Build history of the part. All positions in model axes, mm. Face numbers are marked on the shaded views. A direction names the side the tool comes from. Give positions to 0.01 mm unless a question says otherwise; leave off trailing zeros. Order: outer loops, then holes, each group sorted by start corner. A loop starts at its lowest first (then second) coordinate and runs counter-clockwise, first axis right, second up. Notation, with made-up numbers: (87, 74) -> (101, 74) arc R35 ccw to (101, 109) -> close; hole circle Ø10 at (8, -4.5). An arc over 180 degrees is marked (long way). One line per item, written item: value. Start each with the question number.
(1) Saw through at B-B on x = -90. Give the cut face in (y, z), plus the area to 3 significant figures.
(2) Two-plate mould, pull along Y, no slides. Class the marked faces 6, 7, 8 and 9: +Y half, -Y half, draft (parallel to the pull), parting line (faces both ways), or undercut.
(3) Probe line 1 (X direction, y = 27, z = 10.5) (3 decimals); line 2 (Z direction, x = 103, y = 25); line 3 (X direction, y = 39, z = 26.5). List the from-to ranges inside material, lowest first.
(4) Which spindle directions (+Z, -Z, +X, -X, +Y, -Y) get a long thin tool onto all of the face, cutting with end or side? Do the marked faces 1, 2, 3, 4 and 5. Say none if no direction does.
(5) Saw through at C-C on z = 4.5. Give the cut face in (x, y) (3 decimals).
(6) Pin check, flat tips, straight feed: pin 1 (12 mm diameter, centred on x = 37.5, z = 19, fed in from +Y); pin 2 (14.5 mm diameter, centred on x = 111.5, z = -3.5, fed in from -Y); pin 3 (1.5 mm diameter, centred on y = 27, z = 14.5, fed in from +X) (3 decimals); pin 4 (2 mm diameter, centred on y = 44.5, z = -3, fed in from -X) (3 decimals). Stop position of each tip, or through.
(7) Saw through at A-A on z = -12.5. Give the cut face in (x, y) (3 decimals), plus the area to 3 significant figures.
```python
from build123d import *

# Parameters (mm, degrees)
BOSS_EXTRUDE2_DEPTH             = 120.9
BOSS_EXTRUDE1_REACH             = 138.078
SKETCH2_W                       = 18.2
SKETCH2_H                       = 43.65
BOSS_EXTRUDE1_DIRECTION_2_DEPTH = 18
M6_CLEARANCE_HOLE1_D            = 6.4
CUT_EXTRUDE6_DEPTH              = 137.078193862
CUT_EXTRUDE6_DEPTH_BACK         = 137.078193862
SKETCH13_W                      = 145
SKETCH13_H                      = 13.5
SKETCH13_W_2                    = 161.8
SKETCH13_H_2                    = 14
CHAMFER5_SIZE                   = 4.823085464
CHAMFER5_SIZE_2                 = 18
CHAMFER6_SIZE                   = 18
CHAMFER6_SIZE2                  = 4.823085464
CHAMFER7_SIZE                   = 7
CHAMFER7_SIZE_2                 = 10.646755418
CUT_EXTRUDE8_REACH              = 131.701
SKETCH15_W                      = 10
SKETCH15_H                      = 6
FILLET2_R                       = 20


with BuildPart() as part:
    # Sketch1 → Boss-Extrude2 (new, symmetric)
    with BuildSketch(Plane(origin=(0, 0, 0), x_dir=(0, 0, -1), z_dir=(1, 0, 0))):
        Polygon((0, 0), (-29.329393675, 50.8), (-36.329393675, 50.8), (-36.329393675, 13.8), (-6.735198172, 0), align=None)
    extrude(amount=BOSS_EXTRUDE2_DEPTH, both=True)

    # Boss-Extrude1: up to this plane
    boss_extrude1_end = Plane(origin=(120.9, 0, 0), z_dir=(0, -0.5000000000000043, 0.8660254037844363))
    # Sketch2 → Boss-Extrude1 (add, up to the surface)
    with BuildSketch(Plane.XY, mode=Mode.PRIVATE) as boss_extrude1_sk1:
        with Locations((108.175, 25.4)):
            Rectangle(SKETCH2_W, SKETCH2_H)
    boss_extrude1_tool1 = split(extrude(boss_extrude1_sk1.sketch, amount=BOSS_EXTRUDE1_REACH, mode=Mode.PRIVATE), bisect_by=boss_extrude1_end, keep=Keep.BOTH, mode=Mode.PRIVATE)
    add(boss_extrude1_tool1.solids().sort_by_distance((108.175, 25.4, 0))[0])
    # Sketch2 → Boss-Extrude1 (add, up to the surface)
    with BuildSketch(Plane.XY, mode=Mode.PRIVATE) as boss_extrude1_sk2:
        with Locations((-108.175, 25.4)):
            Rectangle(SKETCH2_W, SKETCH2_H)
    boss_extrude1_tool2 = split(extrude(boss_extrude1_sk2.sketch, amount=BOSS_EXTRUDE1_REACH, mode=Mode.PRIVATE), bisect_by=boss_extrude1_end, keep=Keep.BOTH, mode=Mode.PRIVATE)
    add(boss_extrude1_tool2.solids().sort_by_distance((-108.175, 25.4, 0))[0])

    # Sketch2 → Boss-Extrude1 direction 2 (add)
    with BuildSketch(Plane.XY):
        with Locations((108.175, 25.4)):
            Rectangle(SKETCH2_W, SKETCH2_H)
        with Locations((-108.175, 25.4)):
            Rectangle(SKETCH2_W, SKETCH2_H)
    extrude(amount=-BOSS_EXTRUDE1_DIRECTION_2_DEPTH)

    # M6 Clearance Hole1 (through all)
    with Locations(Plane(origin=(117.275, 0, 0), x_dir=(0, 0, -1), z_dir=(1, 0, 0))):
        with Locations((2.420606325, 25.4)):
            Hole(M6_CLEARANCE_HOLE1_D / 2)

    # Sketch13 → Cut-Extrude6 (cut, two sides: drawn at the far end of the back side and taken through both)
    with BuildSketch(Plane.XY.offset(-CUT_EXTRUDE6_DEPTH_BACK)):
        with Locations((0, 6.75)):
            Rectangle(SKETCH13_W, SKETCH13_H)
        with Locations((0, 30.8)):
            Rectangle(SKETCH13_W_2, SKETCH13_H_2)
    extrude(amount=CUT_EXTRUDE6_DEPTH + CUT_EXTRUDE6_DEPTH_BACK, mode=Mode.SUBTRACT)

    # Chamfer5
    # the kernel refuses this chamfer: 18, 4.823085464 mm, written as the material it takes off along each edge
    with BuildSketch(Plane(origin=(80.9, 37.8, 21.823840175), x_dir=(0, 0.9306108519370808, 0.366010166876469), z_dir=(-1, 0, 0))) as chamfer5_piece_1:
        Polygon((CHAMFER5_SIZE * 0.988937722204, -CHAMFER5_SIZE * 0.148331323403), (CHAMFER5_SIZE_2 * 0.366010166876, -CHAMFER5_SIZE_2 * 0.930610851937), (0, 0), align=None)
    extrude(amount=161.8, mode=Mode.SUBTRACT)

    # Chamfer6
    chamfer6_edges = [part.edges().sort_by_distance(p)[0] for p in [
        (0, 23.8, 36.329393675),
    ]]
    chamfer6_side = [part.faces().sort_by_distance(p)[0] for p in [
        (0, 23.8, 25.035165041),
    ]]
    chamfer(chamfer6_edges, length=CHAMFER6_SIZE, length2=CHAMFER6_SIZE2, reference=chamfer6_side[0])

    # Chamfer7
    # the kernel refuses this chamfer: 10.646755418, 7 mm, written as the material it takes off along each edge
    with BuildSketch(Plane(origin=(148.485482138, 13.8, 36.329393675), x_dir=(0, 0.9993026620124821, 0.037338849671180216), z_dir=(-1, 0, 0))) as chamfer7_piece_1:
        Polygon((CHAMFER7_SIZE * 0.999302662012, CHAMFER7_SIZE * 0.0373388496712), (-CHAMFER7_SIZE_2 * 0.456164044176, CHAMFER7_SIZE_2 * 0.88989570442), (0, 0), align=None)
    extrude(amount=296.970964275, mode=Mode.SUBTRACT)

    # Cut-Extrude8: up to this plane
    cut_extrude8_end = Plane(origin=(-80.9, 23.8, 18.329393675), z_dir=(0, -0.965925826289069, -0.25881904510251824))
    # Sketch15 → Cut-Extrude8 (cut, up to the surface)
    with BuildSketch(Plane(origin=(0, 13.5, 7.794228634), x_dir=(-1, 0, 0), z_dir=(0, 0.8660254037844363, 0.5000000000000042)), mode=Mode.PRIVATE) as cut_extrude8_sk1:
        with Locations((-50, 3)):
            Rectangle(SKETCH15_W, SKETCH15_H)
    cut_extrude8_tool1 = split(extrude(cut_extrude8_sk1.sketch, amount=CUT_EXTRUDE8_REACH, mode=Mode.PRIVATE), bisect_by=cut_extrude8_end, keep=Keep.BOTH, mode=Mode.PRIVATE)
    add(cut_extrude8_tool1.solids().sort_by_distance((50, 12, 10.392305))[0], mode=Mode.SUBTRACT)
    # Sketch15 → Cut-Extrude8 (cut, up to the surface)
    with BuildSketch(Plane(origin=(0, 13.5, 7.794228634), x_dir=(-1, 0, 0), z_dir=(0, 0.8660254037844363, 0.5000000000000042)), mode=Mode.PRIVATE) as cut_extrude8_sk2:
        with Locations((50, 3)):
            Rectangle(SKETCH15_W, SKETCH15_H)
    cut_extrude8_tool2 = split(extrude(cut_extrude8_sk2.sketch, amount=CUT_EXTRUDE8_REACH, mode=Mode.PRIVATE), bisect_by=cut_extrude8_end, keep=Keep.BOTH, mode=Mode.PRIVATE)
    add(cut_extrude8_tool2.solids().sort_by_distance((-50, 12, 10.392305))[0], mode=Mode.SUBTRACT)

    # Fillet1
    # an asymmetric fillet: 4, 1 mm, written as the material it takes off along each edge
    with BuildSketch(Plane(origin=(80.9, 38.736334118, 36.329393675), x_dir=(0, 1, 0), z_dir=(-1, 0, 0))) as fillet1_piece_1:
        with BuildLine():
            Bezier((2.10707295, 0), (0, 0), (1.141147124, 4.258819045), weights=[1, 0.608761429, 1])
            Line((1.141147124, 4.258819045), (0, 0))
            Line((0, 0), (2.10707295, 0))
        make_face()
    extrude(amount=161.8, mode=Mode.SUBTRACT)

    # Fillet2
    fillet2_edges = [part.edges().sort_by_distance(p)[0] for p in [
        (-96.7, 0, 6.735198172),
        (96.7, 0, 6.735198172),
    ]]
    fillet(fillet2_edges, radius=FILLET2_R)


solid = part.part
```
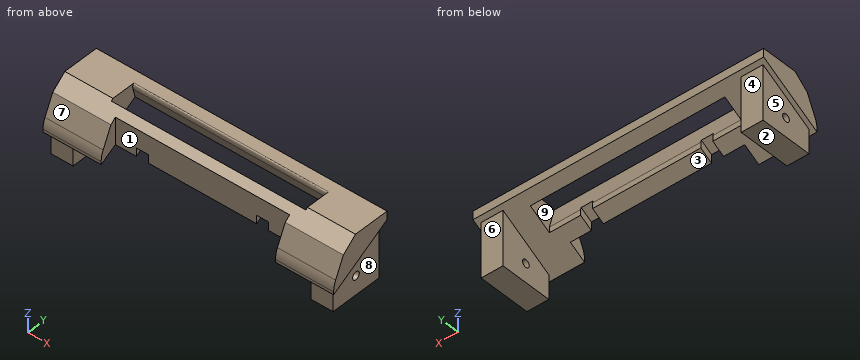
Results below:
1. outline: (0, 0) -> (50.8, 29.33) -> (50.8, 36.33) -> (20.8, 36.33) -> (9.3, 26.68) -> (1.87, 10.75) arc R20 ccw to (0, 2.3) -> close
1. area: 861 mm²
2. face 6: +Y half
2. face 7: -Y half
2. face 8: draft
2. face 9: undercut
3. line 1: x = -117.275 to -99.075, 99.075 to 117.275
3. line 2: z = -18 to -5.6, 0.75 to 36.33
3. line 3: x = -120.9 to -80.9, 80.9 to 120.9
4. face 1: +Z, -Z, -Y
4. face 2: -Z, +X, -X, +Y, -Y
4. face 3: -Z, +Y
4. face 4: -Z, +X, -X, +Y
4. face 5: -Z, -X, +Y
5. outline: (-120.9, 0.121) -> (-72.5, 0.121) -> (-72.5, 7.794) -> (-99.075, 7.794) -> (-99.075, 47.225) -> (-117.275, 47.225) -> (-117.275, 7.794) -> (-120.9, 7.794) -> close; (72.5, 0.121) -> (120.9, 0.121) -> (120.9, 7.794) -> (117.275, 7.794) -> (117.275, 47.225) -> (99.075, 47.225) -> (99.075, 7.794) -> (72.5, 7.794) -> close
6. pin 1: stops at y = 43.3
6. pin 2: stops at y = 0
6. pin 3: stops at x = 117.275
6. pin 4: stops at x = -117.275
7. outline: (-117.275, 3.575) -> (-99.075, 3.575) -> (-99.075, 47.225) -> (-117.275, 47.225) -> close; (99.075, 3.575) -> (117.275, 3.575) -> (117.275, 47.225) -> (99.075, 47.225) -> close
7. area: 1,590 mm²
